Geometry: final body of the model. Coordinates: model frame, mm. A direction names the side the tool comes from. Round coordinates to 2 decimals unless told otherwise and drop trailing zeros. Loops run counter-clockwise (first coordinate to the right, second up) from the corner with the lowest first, then second, coordinate; pieces in that order, holes last. Notation, with made-up numbers: M -8,-17.5 L 38,-17.5 A27 cw 38,1.5 Z; hole C -39,83.25 d2. An arc over 180 degrees is marked long. Write each question's results on one line, items separated by ' | '.
```python
from build123d import *
from build123d.topology import SkipClean

# Parameters (mm, degrees)
SKETCH1_R           = 34.5
BOSS_EXTRUDE1_DEPTH = 24
SKETCH6_R           = 1.5
CUT_EXTRUDE6_DEPTH  = 24
CUT_EXTRUDE7_DEPTH  = 24
CIRPATTERN1_COUNT   = 6


with BuildPart() as part:
    # Sketch1 → Boss-Extrude1 (new body)
    with BuildSketch(Plane(origin=(0, 0, 0), x_dir=(1, 0, 0), z_dir=(0, 1, 0))):
        with Locations(Location((0, 0, 0), (0, 0, 270))):
            Circle(SKETCH1_R)
    extrude(amount=BOSS_EXTRUDE1_DEPTH)

    # Sketch6 → Cut-Extrude6 (cut)
    with BuildSketch(Plane(origin=(0, 0, 0), x_dir=(1, 0, 0), z_dir=(0, 1, 0))):
        with Locations(Location((0, 0, 0), (0, 0, 90))):
            Circle(SKETCH6_R)
    extrude(amount=CUT_EXTRUDE6_DEPTH, mode=Mode.SUBTRACT)

    # Sketch3 → Cut-Extrude7 (cut)
    with BuildSketch(Plane(origin=(0, 0, 0), x_dir=(1, 0, 0), z_dir=(0, 1, 0))):
        with BuildLine():
            ThreePointArc((4.03179755, 10.82025609), (4.919774713, 10.446489846), (5.773502692, 10))
            Line((5.773502692, 10), (22.209007182, 10))
            ThreePointArc((22.209007182, 10), (26.624465103, 12.65399673), (26.352478671, 17.798507463))
            ThreePointArc((26.352478671, 17.798507463), (21.242536942, 23.664205549), (14.861330114, 28.113713153))
            ThreePointArc((14.861330114, 28.113713153), (11.140652369, 28.497958465), (8.19451597, 26.193318003))
            Line((8.19451597, 26.193318003), (2.222782323, 15.849971917))
            ThreePointArc((2.222782323, 15.849971917), (1.960414336, 12.915429114), (4.03179755, 10.82025609))
        make_face()
    cut_extrude7 = extrude(amount=CUT_EXTRUDE7_DEPTH, mode=Mode.SUBTRACT)

    # CirPattern1: Cut-Extrude7 ×6 about axis
    cirpattern1_axis = Axis((0, 0, 0), (0, 1, 0))
    for i in range(1, CIRPATTERN1_COUNT):
        add(cut_extrude7.rotate(cirpattern1_axis, i * 360 / CIRPATTERN1_COUNT), mode=Mode.SUBTRACT)

    # Sketch14 → Revolve1 (revolve)
    with BuildSketch(Plane.XY):
        Polygon((32, 13), (32, 12), (34.5, 12), (34.5, 14), align=None)
    revolve1 = revolve(axis=Axis((0, 24, 0), (0, -1, 0)))

    # Mirror11: Revolve1 across plane
    add(revolve1.mirror(Plane.ZX.offset(12)))

    # Sketch15 → Cut-Revolve5 (revolve, cut)
    with SkipClean():  # the faces are left unmerged after this step: merging them gives an invalid solid
        with BuildSketch(Plane.XY, mode=Mode.PRIVATE) as cut_revolve5_sk:
            Polygon((1.5, 6), (1.5, 0), (0, 0), (0, 6), (0, 24), (31.8, 24), (31.8, 10), (27.8, 6), align=None)
        revolve(cut_revolve5_sk.sketch.rotate(Axis((0, 6, 0), (0, -1, 0)), 270), axis=Axis((0, 6, 0), (0, -1, 0)), mode=Mode.SUBTRACT)


solid = part.part
```
1. Section A-A (y = 22.5). Output: boundary loops of the cut face in (x, z), then the cut area to 3 significant figures.
Answer key:
outline: C 0,0 d69; hole C 0,0 d63.6 | area: 562 mm²
2. Section B-B (z = -12.5). Count the separate pieces of the cut face and the enclosed holes in it, then the cut area to 3 significant figures.
Answer key:
separate pieces: 4 | enclosed holes: 0 | area: 230 mm²
3. Ray query, probe 1 along Y at (x, z) = (-0.5, -7.5); probe 2 along Z at (x, y) = (9, 5.75); probe 3 along Z at (x, y) = (5.5, 1.75). Return the intervals inside material, ascending.
Answer key:
probe 1: y = 0 to 6 | probe 2: z = -33.31 to -27.24, -10 to 8.15, 30.5 to 33.31 | probe 3: z = -34.06 to -21.53, -10.15 to 10.47, 31.32 to 34.06
4. Access query for faces 1 (the face through (22.564, 8.416, 20.097)), 2 (the face through (15.64, 2.96, 15.09)). Directions: +Z, -Z, +X, -X, +Y, -Y. A direction counts if a zero-diameter tool reaches every point of the face in a straight line with its end or side. Return the directions, or none.
Answer key:
face 1: +Y | face 2: +Y, -Y
5. Pin query (flat end, axial travel): P1, Ø1.8, axis at x = 12.5, y = 2.5, coming from the -Z side; P2, Ø5, axis at x = 16, y = 9, coming from the +Z side; P3, Ø10, axis at y = 13, z = -27.5, coming from the -X side; P4, Ø2, axis at x = 4.5, z = 10.5, coming from the -Y side. Return the tip coordinate at first contact, or that it passes through.
Answer key:
P1: stops at z = -32.49 | P2: stops at z = 31.75 | P3: stops at x = -26.15 | P4: stops at y = 0
